```python
from build123d import *

# Parameters (mm, degrees)
SKETCH_1_W          = 20
SKETCH_1_H          = 5
EXTRUDE_1_DEPTH     = 35
SKETCH_2_W          = 30
SKETCH_2_H          = 20
EXTRUDE_2_DEPTH     = 3
FILLET_1_R          = 2
FILLET_2_R          = 2
FILLET_3_R          = 2
FILLET_4_R          = 2
SKETCH_4_W          = 30
SKETCH_4_H          = 40
EXTRUDE_3_DEPTH     = 2.5
FILLET_5_R          = 2
FILLET_6_R          = 2
CUT_EXTRUDE_2_DEPTH = 3
SKETCH_6_R          = 1.475
SKETCH_6_R_2        = 1.95
SKETCH_6_R_3        = 2.425
CUT_EXTRUDE_3_DEPTH = 3
SKETCH_8_W          = 3
SKETCH_8_H          = 7.5
CUT_EXTRUDE_4_DEPTH = 30


with BuildPart() as part:
    # 草图1 → 凸台-拉伸1 (new body)
    with BuildSketch(Plane(origin=(0, 0, 0), x_dir=(0, 0, -1), z_dir=(1, 0, 0))):
        Rectangle(SKETCH_1_W, SKETCH_1_H)
    extrude(amount=-EXTRUDE_1_DEPTH)

    # 草图2 → 凸台-拉伸2 (add)
    with BuildSketch(Plane(origin=(0, 0, 0), x_dir=(0, 0, -1), z_dir=(1, 0, 0))):
        Rectangle(SKETCH_2_W, SKETCH_2_H)
    extrude(amount=EXTRUDE_2_DEPTH)

    # 圆角1
    fillet_1_edges = [part.edges().sort_by_distance(p)[0] for p in [
        (1.5, 10, -15),
    ]]
    fillet(fillet_1_edges, radius=FILLET_1_R)

    # 圆角2
    fillet_2_edges = [part.edges().sort_by_distance(p)[0] for p in [
        (1.5, 10, 15),
    ]]
    fillet(fillet_2_edges, radius=FILLET_2_R)

    # 圆角3
    fillet_3_edges = [part.edges().sort_by_distance(p)[0] for p in [
        (1.5, -10, -15),
    ]]
    fillet(fillet_3_edges, radius=FILLET_3_R)

    # 圆角4
    fillet_4_edges = [part.edges().sort_by_distance(p)[0] for p in [
        (1.5, -10, 15),
    ]]
    fillet(fillet_4_edges, radius=FILLET_4_R)

    # 草图4 → 凸台-拉伸3 (add, symmetric)
    with BuildSketch(Plane(origin=(0, 0, 0), x_dir=(1, 0, 0), z_dir=(0, 1, 0))):
        with Locations((-20, 0)):
            Rectangle(SKETCH_4_W, SKETCH_4_H)
    extrude(amount=EXTRUDE_3_DEPTH, both=True)

    # 圆角5
    fillet_5_edges = [part.edges().sort_by_distance(p)[0] for p in [
        (-5, 0, -10),
    ]]
    fillet(fillet_5_edges, radius=FILLET_5_R)

    # 圆角6
    fillet_6_edges = [part.edges().sort_by_distance(p)[0] for p in [
        (-5, 0, 10),
    ]]
    fillet(fillet_6_edges, radius=FILLET_6_R)

    # 草图5 → 切除-拉伸2 (cut)
    with BuildSketch(Plane(origin=(0, 0, 0), x_dir=(0, 0, -1), z_dir=(1, 0, 0))):
        with BuildLine():
            Line((-12, -1.5), (-15, -1.5))
            Line((-15, -1.5), (-15, 1.5))
            Line((-15, 1.5), (-12, 1.5))
            ThreePointArc((-12, 1.5), (-10.5, 0), (-12, -1.5))
        make_face()
        with BuildLine():
            Line((12, 1.5), (15, 1.5))
            Line((15, 1.5), (15, -1.5))
            Line((15, -1.5), (12, -1.5))
            ThreePointArc((12, -1.5), (10.5, 0), (12, 1.5))
        make_face()
    extrude(amount=CUT_EXTRUDE_2_DEPTH, mode=Mode.SUBTRACT)

    # 草图6 → 切除-拉伸3 (cut)
    with BuildSketch(Plane(origin=(0, 0, 0), x_dir=(0, 0, -1), z_dir=(1, 0, 0))):
        with Locations((0, -7)):
            Circle(SKETCH_6_R)
        with Locations((-7, -7)):
            Circle(SKETCH_6_R_2)
        with Locations((7, -7)):
            Circle(SKETCH_6_R_3)
        with Locations(Location((7, 7, 0), (0, 0, 180))):
            Circle(SKETCH_6_R_3)
        with Locations(Location((0, 7, 0), (0, 0, 180))):
            Circle(SKETCH_6_R)
        with Locations(Location((-7, 7, 0), (0, 0, 180))):
            Circle(SKETCH_6_R_2)
    extrude(amount=CUT_EXTRUDE_3_DEPTH, mode=Mode.SUBTRACT)

    # 草图8 → 切除-拉伸4 (cut)
    with BuildSketch(Plane(origin=(0, 0, -15), x_dir=(-1, 0, 0), z_dir=(0, 0, -1))):
        with Locations((-1.5, -6.25)):
            Rectangle(SKETCH_8_W, SKETCH_8_H)
    extrude(amount=-CUT_EXTRUDE_4_DEPTH, mode=Mode.SUBTRACT)


solid = part.part
```
Input: part model. Units: mm. Frame: model coordinates. A direction names the side the tool comes from. Give positions to 0.01 mm unless a question says otherwise; leave off trailing zeros. Write each loop counter-clockwise with the first axis right and the second up, starting at its lowest first coordinate (ties: lowest second). Pieces come first, ordered by that corner, then holes. Notation, with made-up numbers: (46.5, -20) - (98.5, -20) arc R13 ccw to (98.5, 1) - close; hole circle Ø5 at (6, 48.25). An arc over 180 degrees is marked (long way). Write item = value, one per line. Start each with the question number.
1) Cut plane D-D (y = 0). Return loops of the section in (x, z).
2) Pin query (flat end, axial travel): pin 1 (1.1 mm diameter, centred on x = 1, y = -2, fed in from -Z); pin 2 (2.5 mm diameter, centred on x = -1.5, y = 0, fed in from -Z); pin 3 (1.5 mm diameter, centred on y = -0.5, z = -14.5, fed in from +X). Return the tip coordinate at first contact, or that it passes through.
3) Cut plane C-C (z = -12.5). Return loops of the section in (x, y), and give its area (4 significant figures).
4) Material intervals for L1, parallel to Z at x = 0.8, y = 7 (3 decimals); L2, parallel to Y at x = 1.1, z = 7; L3, parallel to Y at x = 2.25, z = 0 (3 decimals), sorted ascending. Write a range as [from, to].
5) Reachability of faces 1 (the face through (1.5, 0, -10.5)), 2 (the face through (-5, 0, 16)), 3 (the face through (1, -2, 15)), 4 (the face through (-18, 2.5, 0)), 5 (the face through (1, -2, -15)) from +Z, -Z, +X, -X, +Y, -Y: full face, straight path, thin tool, end or side. Return the list, or none.
6) Cut plane B-B (y = 7). Return loops of the section in (x, z) (3 decimals).
7) Draft query along X for faces 6 (the face through (-35, 0, 0)), 7 (the face through (-5, 0, -16)), 8 (the face through (1.48, 8.48, -8.92)). Return one class per face: pulls with the +X half, pulls with the -X half, needs draft (parallel to the pull), parting line crosses it, or undercut.
8) Cut plane A-A (z = 7). Return loops of the section in (x, y), and give its area (3 significant figures).
Answers follow:
q1.outline = (-35, -20) - (-5, -20) - (-5, -12) arc R2 cw to (-3, -10) - (0, -10) - (0, -10.5) - (3, -10.5) - (3, 10.5) - (0, 10.5) - (0, 10) - (-3, 10) arc R2 cw to (-5, 12) - (-5, 20) - (-35, 20) - close
q2.pin_1 = -15
q2.pin_2 = -10
q2.pin_3 = -5
q3.outline = (-35, -2.5) - (-5, -2.5) - (-5, 2.5) - (-35, 2.5) - close; (0, -2.5) - (3, -2.5) - (3, -1.5) - (0, -1.5) - close; (0, 1.5) - (3, 1.5) - (3, 10) - (0, 10) - close
q3.area = 178.5 mm^2
q4.L1 = [-15, -9.425], [-4.575, -1.475], [1.475, 5.05], [8.95, 15]
q4.L2 = [-2.5, 5.05], [8.95, 10]
q4.L3 = [-2.5, 5.525], [8.475, 10]
q5.face_1 = -Z, +X
q5.face_2 = +Z, +Y, -Y
q5.face_3 = +Z, +X, +Y, -Y
q5.face_4 = +Z, -Z, -X, +Y
q5.face_5 = -Z, +X, +Y, -Y
q6.outline = (0, -15) - (3, -15) - (3, -9.425) - (0, -9.425) - close; (0, -4.575) - (3, -4.575) - (3, -1.475) - (0, -1.475) - close; (0, 1.475) - (3, 1.475) - (3, 5.05) - (0, 5.05) - close; (0, 8.95) - (3, 8.95) - (3, 15) - (0, 15) - close
q7.face_6 = pulls with the -X half
q7.face_7 = undercut
q7.face_8 = needs draft
q8.outline = (-35, -2.5) - (3, -2.5) - (3, 5.05) - (0, 5.05) - (0, 2.5) - (-35, 2.5) - close; (0, 8.95) - (3, 8.95) - (3, 10) - (0, 10) - close
q8.area = 201 mm^2
